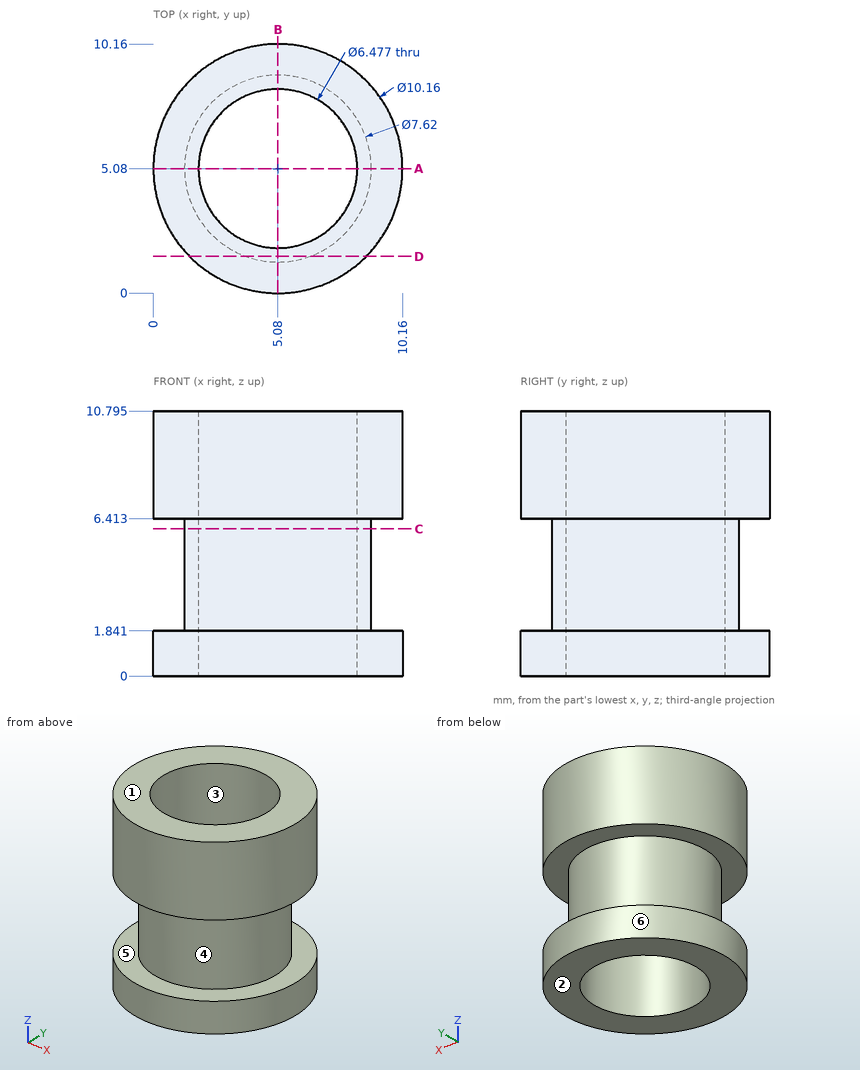
Geometry: see drawing. Coordinates: mm, zero at the bounding-box minimum. A direction names the side the tool comes from. Coordinates: 2 decimals unless noted, no trailing zeros. Write each loop counter-clockwise with the first axis right and the second up, starting at its lowest first coordinate (ties: lowest second). Pieces come first, ordered by that corner, then holes.
1) Mould query, pull axis Z, two halves, no side actions, for the marked faces 1, 2, 3 and 4. Classes: pulls with the +Z half, pulls with the -Z half, needs draft (parallel to the pull), parting line crosses it, or undercut.
2) Section A-A on y = 5.08. Output: boundary loops of the cut face in (x, z) (1 decimal).
3) Section D-D on y = 1.5. Output: boundary loops of the cut face in (x, z) (1 decimal).
4) Set-up query: the marked faces 5 and 6. Return all of +Z, -Z, +X, -X, +Y, -Y with unobstructed straight access to the full face (end or side cutting, diameter ignored); none if empty.
5) Pin query (flat end, axial travel): pin 1 Ø1.5 at (x, z) = (7.5, 6.5) entering from +Y; pin 2 Ø3 at (x, z) = (6, 6.5) entering from -Y; pin 3 Ø5 at (x, y) = (5.08, 5.08) entering from -Z; pin 4 Ø2 at (x, z) = (4, 4) entering from -Y. Return the tip coordinate at first contact, or that it passes through.
6) Section C-C on z = 6. Output: boundary loops of the cut face in (x, y).
7) Material intervals for line 1 along Z through (x, y) = (6.25, 0.75) (1 decimal); line 2 along Y through (x, z) = (5.08, 3); line 3 along X through (y, z) = (7, 2.5), sorted ascending.
Check result:
1. face 1: pulls with the +Z half
1. face 2: pulls with the -Z half
1. face 3: needs draft
1. face 4: undercut
2. outline: (0, 0) - (1.8, 0) - (1.8, 10.8) - (0, 10.8) - (0, 6.4) - (1.3, 6.4) - (1.3, 1.8) - (0, 1.8) - close; (8.3, 0) - (10.2, 0) - (10.2, 1.8) - (8.9, 1.8) - (8.9, 6.4) - (10.2, 6.4) - (10.2, 10.8) - (8.3, 10.8) - close
3. outline: (1.5, 0) - (8.7, 0) - (8.7, 1.8) - (6.4, 1.8) - (6.4, 6.4) - (8.7, 6.4) - (8.7, 10.8) - (1.5, 10.8) - (1.5, 6.4) - (3.8, 6.4) - (3.8, 1.8) - (1.5, 1.8) - close
4. face 5: none
4. face 6: +Z, -Z
5. pin 1: stops at y = 9.88
5. pin 2: stops at y = 0
5. pin 3: passes through
5. pin 4: stops at y = 1.27
6. outline: circle Ø7.62 at (5.08, 5.08); hole circle Ø6.48 at (5.08, 5.08)
7. line 1: z = 0 to 1.8, 6.4 to 10.8
7. line 2: y = 1.27 to 1.84, 8.32 to 8.89
7. line 3: x = 1.79 to 2.47, 7.69 to 8.37
